Read the model definition and answer for the solid it produces. Units are mm, in the model's axes. Round coordinates to 2 decimals unless told otherwise and drop trailing zeros. Loops run counter-clockwise (first coordinate to the right, second up) from the corner with the lowest first, then second, coordinate; pieces in that order, holes last. Notation, with made-up numbers: (20, -5.5) - (60, -5.5) arc R22 cw to (60, 12.5) - close; hole circle Ø10 at (49, 37). An arc over 180 degrees is marked (long way). Use CSV: the item, a comma, the result in double quotes. Start each with the question number.
1. Find section B-B (z = 0). Give the vertices of the cut face in (x, y).
2. Find section A-A (x = 0). Give the vertices of the cut face in (y, z), and give its area (3 significant figures).
3. Consider line 1 along X through (y, z) = (12, 0); line 2 along Y through (x, z) = (-3, -7.5); line 3 along X through (y, z) = (16, -6). Determine where each line is inside the solid, lowest interval first.
4. Find section C-C (y = 5). Give the vertices of the cut face in (x, z), and give its area (3 significant figures).
5. Determine the mould class of faces 1 (the flat face through (5, -12.7, 0)), 2 (the conical face through (16, -18, -4)), 3 (the cylindrical face through (26.36, 0.18, -5.85)) for opening direction Z: +Z half, -Z half, draft (parallel to the pull), parting line (faces both ways), or undercut.
6. Given pin 1 Ø4 at (y, z) = (9, 19) entering from +X; pin 2 Ø24 at (x, z) = (3.5, 1.5) entering from -Y; pin 3 Ø9 at (x, z) = (0, 0) entering from -Y, each flat-ended and moving along its own axis, determine where each tip first touches the part or whether it passes through.
from build123d import *

# Parameters (mm, degrees)
SKETCH2_R          = 4
CUT_EXTRUDE1_DEPTH = 54.356


with BuildPart() as part:
    # Sketch1 → Revolve3 (revolve)
    with BuildSketch(Plane.XY, mode=Mode.PRIVATE) as revolve3_sk:
        with BuildLine():
            Line((0, 12.7), (0, -12.7))
            Line((0, -12.7), (11, -12.7))
            Line((11, -12.7), (11, -12.919434808))
            ThreePointArc((11, -12.919434808), (12.487804595, -16.511444297), (16.079737075, -17.999434801))
            Line((16.079737075, -17.999434801), (21.919737075, -17.999737061))
            ThreePointArc((21.919737075, -17.999737061), (25.512009489, -16.511932473), (27, -12.919737068))
            Line((27, -12.919737068), (27, 12.919737068))
            ThreePointArc((27, 12.919737068), (25.512009489, 16.511932473), (21.919737075, 17.999737061))
            Line((21.919737075, 17.999737061), (16.079737075, 17.999434801))
            ThreePointArc((16.079737075, 17.999434801), (12.487804595, 16.511444297), (11, 12.919434808))
            Line((11, 12.919434808), (11, 12.7))
            Line((11, 12.7), (0, 12.7))
        make_face()
    revolve(revolve3_sk.sketch.rotate(Axis((0, 12.7, 0), (0, -1, 0)), 90), axis=Axis((0, 12.7, 0), (0, -1, 0)))

    # Sketch2 → Cut-Extrude1 (cut)
    with BuildSketch(Plane.XZ.offset(12.7)):
        with Locations(Location((0, 0, 0), (0, 0, 270))):
            Circle(SKETCH2_R)
    extrude(amount=-CUT_EXTRUDE1_DEPTH, mode=Mode.SUBTRACT)


solid = part.part
Filled sheet:
1,outline,"(-27, -12.92) arc R5.08 ccw to (-21.92, -18) - (-16.08, -18) arc R5.08 ccw to (-11, -12.92) - (-11, -12.7) - (-4, -12.7) - (-4, 12.7) - (-11, 12.7) - (-11, 12.92) arc R5.08 ccw to (-16.08, 18) - (-21.92, 18) arc R5.08 ccw to (-27, 12.92) - close; (4, -12.7) - (11, -12.7) - (11, -12.92) arc R5.08 ccw to (16.08, -18) - (21.92, -18) arc R5.08 ccw to (27, -12.92) - (27, 12.92) arc R5.08 ccw to (21.92, 18) - (16.08, 18) arc R5.08 ccw to (11, 12.92) - (11, 12.7) - (4, 12.7) - close"
2,outline,"(-18, -21.92) arc R5.08 ccw to (-12.92, -27) - (12.92, -27) arc R5.08 ccw to (18, -21.92) - (18, -16.08) arc R5.08 ccw to (12.92, -11) - (12.7, -11) - (12.7, -4) - (-12.7, -4) - (-12.7, -11) - (-12.92, -11) arc R5.08 ccw to (-18, -16.08) - close; (-18, 16.08) arc R5.08 ccw to (-12.92, 11) - (-12.7, 11) - (-12.7, 4) - (12.7, 4) - (12.7, 11) - (12.92, 11) arc R5.08 ccw to (18, 16.08) - (18, 21.92) arc R5.08 ccw to (12.92, 27) - (-12.92, 27) arc R5.08 ccw to (-18, 21.92) - close"
2,area,"1,460 mm²"
3,line 1,"x = -27 to -4, 4 to 27"
3,line 2,"y = -12.7 to 12.7"
3,line 3,"x = -25.26 to -10.44, 10.44 to 25.26"
4,outline,"circle Ø54 at (0, 0); hole circle Ø8 at (0, 0)"
4,area,"2,240 mm²"
5,face 1,"undercut"
5,face 2,"draft"
5,face 3,"parting line"
6,pin 1,"stops at x = 20.98"
6,pin 2,"stops at y = -17.99"
6,pin 3,"stops at y = -12.7"
